Autodesk Inventor part; units mm, degrees
ref_plane "YZ Plane" through (0, 0, 0) normal (1, 0, 0) x (0, 1, 0)
ref_plane "XZ Plane" through (0, 0, 0) normal (0, 1, 0) x (-1, 0, 0)
ref_plane "XY Plane" through (0, 0, 0) normal (0, 0, 1) x (1, 0, 0)
sketch "Sketch1" plane through (0, 0, 0) normal (0, 1, 0) x (-1, 0, 0)
  line L0 (0, 0) -> (162, 0)
  line L1 (162, 0) -> (162, -156)
  line L2 (162, -156) -> (0, -156)
  line L3 (0, -156) -> (0, 0)
  dimension "d0" = 162
  dimension "d1" = 156
extrude "Extrusion1" add sketch "Sketch1" along normal blind 6
sketch "Sketch3" plane through (0, 0, 0) normal (1, 0, 0) x (0, 0, -1)
  line L0 (156, 6) -> (0, 6)
  line L1 (0, 6) -> (156, 6)
  line L2 (156, 6) -> (156, 156)
  line L3 (156, 156) -> (0, 156)
  line L4 (0, 156) -> (0, 6)
  point P0 (0, 0)
  dimension "d4" = 150
extrude "Extrusion2" add sketch "Sketch3" against normal blind 6
sketch "Sketch4" plane through (-162, 0, -156) normal (-1, 0, 0) x (0, 0, 1)
  line L0 (0, 6) -> (156, 6)
  line L1 (156, 156) -> (0, 156)
  line L2 (0, 6) -> (156, 6)
  line L3 (156, 6) -> (156, 156)
  line L4 (156, 156) -> (0, 156)
  line L5 (0, 156) -> (0, 6)
  point P0 (156, 0)
extrude "Extrusion3" add sketch "Sketch4" against normal blind 6
sketch "Sketch5" plane through (-162, 156, 0) normal (0, 1, 0) x (1, 0, 0)
  line L0 (0, 156) -> (0, 0)
  line L1 (162, 156) -> (0, 156)
  line L2 (0, 156) -> (0, 0)
  line L3 (0, 0) -> (162, 0)
  line L4 (162, 0) -> (162, 156)
  point P0 (162, 0)
extrude "Extrusion4" add sketch "Sketch5" along normal blind 6
properties part number "Estacion" material "Wood (Cherry)"
The model under review builds one solid part; all positions refer to its coordinate system, in mm. A direction names the side the tool comes from. Round coordinates to 2 decimals unless told otherwise and drop trailing zeros. Loops run counter-clockwise (first coordinate to the right, second up) from the corner with the lowest first, then second, coordinate; pieces in that order, holes last. Notation, with made-up numbers: M -32,-9 L -25,-9 A12 ccw -25,8 Z; hole C 82.25,76.5 d9. An arc over 180 degrees is marked long. Answer as a JSON object with one key per item and string values.
(1) Tool access review of faces 5 (the flat face through (-87, 159, 0)), 6 (the flat face through (-156, 82, -79)): name each direction out of +Z, -Z, +X, -X, +Y, -Y from which nothing blocks a thin tool from reaching the whole face with its end or side.
Resolved:
{"face 5": "+Z, +X, -X, +Y, -Y", "face 6": "+Z, -Z"}
(2) Take a section at C-C on y = 28.5. Give the boundary of the cut face in (x, z), and give its area (3 significant figures).
Resolved:
{"outline": "M -162,-156 L -156,-156 L -156,0 L -162,0 Z; M -6,-156 L 0,-156 L 0,0 L -6,0 Z", "area": "1,870 mm²"}
(3) Draft analysis for pull direction X (two halves, no side actions). For faces 1 (the flat face through (-6, 82, -77)), 2 (the flat face through (-80, 0, -77)), 3 (the flat face through (-162, 80, -79)), 4 (the flat face through (0, 80, -77)), state which applies: released by +X, released by -X, zero draft, split by the parting line, or undercut.
Resolved:
{"face 1": "undercut", "face 2": "zero draft", "face 3": "released by -X", "face 4": "released by +X"}
(4) Take a section at B-B on z = -145.5. Give the boundary of the cut face in (x, y), and give its area (3 significant figures).
Resolved:
{"outline": "M -162,0 L 0,0 L 0,162 L -162,162 Z; hole M -156,6 L -6,6 L -6,156 L -156,156 Z", "area": "3,740 mm²"}
(5) Take a section at A-A on x = -37.5. Give the boundary of the cut face in (y, z).
Resolved:
{"outline": "M 0,-156 L 6,-156 L 6,0 L 0,0 Z; M 156,-156 L 162,-156 L 162,0 L 156,0 Z"}
(6) To check wall thickness, follow line 1 along Y through (x, z) = (-84, -47); line 2 along X through (y, z) = (12.5, -56). State the ranges of each line that lie inside material, in increasing order.
Resolved:
{"line 1": "0 to 6, 156 to 162", "line 2": "-162 to -156, -6 to 0"}
